```python
from build123d import *

# Parameters (mm, degrees)
PAD_DEPTH              = 66
SKETCH001_W            = 31.9
SKETCH001_H            = 39.95
PAD001_DEPTH           = 1
PAD002_DEPTH           = 1.2
PAD003_DEPTH           = 16
SKETCH011_W            = 16.471436
SKETCH011_H            = 30.415474
POCKET_DEPTH           = 5
POCKET001_DEPTH        = 8
POCKET002_DEPTH        = 5
LINEARPATTERN_COUNT    = 2
LINEARPATTERN_PITCH    = 32
POCKET003_DEPTH        = 31.901
LINEARPATTERN001_COUNT = 2
LINEARPATTERN001_PITCH = 28


with BuildPart() as part:
    # Sketch → Pad (new body)
    with BuildSketch(Plane.XY):
        Polygon((14.75, 37.75), (14.75, 0), (-14.75, 0), (-14.75, 37.75), (-12.25, 37.75), (-12.25, 38.75), (-15.95, 38.75), (-15.95, -1.2), (15.95, -1.2), (15.95, 38.75), (12.25, 38.75), (12.25, 37.75), align=None)
    extrude(amount=PAD_DEPTH)

    # Sketch001 (on Face13 of Pad) → Pad001 (join)
    with BuildSketch(Plane(origin=(0, 0, 0), x_dir=(1, 0, 0), z_dir=(0, 0, -1))):
        with Locations((0, -18.775)):
            Rectangle(SKETCH001_W, SKETCH001_H)
    extrude(amount=PAD001_DEPTH)

    # Sketch002 (on Face13 of Pad001) → Pad002 (join)
    with BuildSketch(Plane.XZ.offset(1.2)):
        Polygon((-15.95, 66), (-4, 94), (4, 94), (15.95, 66), align=None)
    extrude(amount=-PAD002_DEPTH)

    # Sketch007 (on Face8 of Pad002) → Pad003 (join)
    with BuildSketch(Plane(origin=(0, 0, 0), x_dir=(-1, 0, 0), z_dir=(0, 1, 0))):
        Polygon((-15.95, 66), (-14.7, 66), (-3.5, 88), (3.5, 88), (14.7, 66), (15.95, 66), (4, 94), (-4, 94), align=None)
    extrude(amount=PAD003_DEPTH)

    # Sketch011 (on Face24 of Pad003) → Pocket (cut)
    with BuildSketch(Plane(origin=(0, 0, -1), x_dir=(1, 0, 0), z_dir=(0, 0, -1))):
        with Locations((0, -31.207737)):
            Rectangle(SKETCH011_W, SKETCH011_H)
    extrude(amount=-POCKET_DEPTH, mode=Mode.SUBTRACT)

    # Sketch012 (on Face33 of Pocket) → Pocket001 (cut)
    with BuildSketch(Plane.XY.offset(94)):
        with BuildLine():
            ThreePointArc((2.985382, 13.549034), (-0.014618, 16.549034), (-3.014618, 13.549034))
            Line((-3.014618, 13.549034), (-3.014618, 11.03404))
            ThreePointArc((-3.014618, 11.03404), (-0.014618, 8.03404), (2.985382, 11.03404))
            Line((2.985382, 13.549034), (2.985382, 11.03404))
        make_face()
    extrude(amount=-POCKET001_DEPTH, mode=Mode.SUBTRACT)

    # Sketch014 (on Face30 of Pocket001) → Pocket002 (cut)
    with BuildSketch(Plane.XZ.offset(1.2)):
        Polygon((0, 25.833173), (-10.237929, 13.747521), (-10.237929, 5.434677), (10.297925, 5.434677), (10.297925, 13.443167), align=None)
    pocket002 = extrude(amount=-POCKET002_DEPTH, mode=Mode.SUBTRACT)

    # LinearPattern: Pocket002 ×2
    with Locations(*[(0, 0, i * LINEARPATTERN_PITCH) for i in range(1, LINEARPATTERN_COUNT)]):
        add(pocket002, mode=Mode.SUBTRACT)

    # Sketch015 (on Face29 of LinearPattern) → Pocket003 (cut, through all)
    with BuildSketch(Plane.YZ.offset(15.95)):
        Polygon((18.770079, 31.374571), (6.687755, 18.189028), (6.687755, 5.829207), (30.620473, 5.829207), (30.620473, 18.442136), align=None)
    pocket003 = extrude(amount=-POCKET003_DEPTH, mode=Mode.SUBTRACT)

    # LinearPattern001: Pocket003 ×2
    with Locations(*[(0, 0, i * LINEARPATTERN001_PITCH) for i in range(1, LINEARPATTERN001_COUNT)]):
        add(pocket003, mode=Mode.SUBTRACT)


solid = part.part
```
Geometry: final body of the model. Coordinates: model frame, mm. A direction names the side the tool comes from. Round coordinates to 2 decimals unless told otherwise and drop trailing zeros. Order: outer loops, then holes, each group sorted by start corner. A loop starts at its lowest first (then second) coordinate and runs counter-clockwise, first axis right, second up. Notation, with made-up numbers: M 44,27 L 51,27 A32 cw 51,60 Z; hole C 82.5,74 d7. An arc over 180 degrees is marked long. Use one line per item in the form item = value. Start each with the question number.
Q1. Cut plane B-B (y = 4). Return loops of the section in (x, z), and give its area (4 significant figures).
Q2. Material intervals for line 1 (X direction, y = 13, z = 58); line 2 (Z direction, x = -13, y = 34.5); line 3 (Y direction, x = -2, z = 75), sorted ascending. Write a range as [from, to].
Q3. Mould query, pull axis Z, two halves, no side actions, for faces 5 (the face through (0, 14, -1)), 6 (the face through (-0.081, 8.035, 91.042)), 7 (the face through (-15.342, 24.778, 52.818)). Classes: +Z half, -Z half, draft (parallel to the pull), parting line (faces both ways), or undercut.
Q4. Cut plane A-A (y = 33.5). Return loops of the section in (x, z), and give its area (3 significant figures).
Q5. Access query for faces 1 (the face through (5.22, -0.61, 51.55)), 2 (the face through (-15.34, 12.81, 24.87)), 3 (the face through (2.66, 14.91, 91.04)), 4 (the face through (9.2, 7.9, 76.8)). Directions: +Z, -Z, +X, -X, +Y, -Y. A direction counts if a zero-diameter tool reaches every point of the face in a straight line with its end or side. Return the directions, or none.
Q6. Pin query (flat end, axial travel): pin 1 Ø3 at (y, z) = (12.5, 91.5) entering from -X; pin 2 Ø4 at (x, y) = (9, 13) entering from +Z; pin 3 Ø2 at (y, z) = (12, 90) entering from +X; pin 4 Ø1.5 at (y, z) = (29.5, 42) entering from +X. Return the tip coordinate at first contact, or that it passes through.
Q7. Cut plane D-D (x = -6). Return loops of the section in (y, z), and give its area (3 significant figures).
Q8. Cut plane C-C (z = 10.5). Return loops of the section in (x, y).
Geometry results:
q1.outline = M -15.95,-1 L 15.95,-1 L 15.95,66 L 4,94 L -4,94 L -15.95,66 Z; hole M -14.75,0 L 14.75,0 L 14.75,66 L 14.7,66 L 3.5,88 L -3.5,88 L -14.7,66 L -14.75,66 Z
q1.area = 348.5 mm^2
q2.line_1 = [-15.95, -14.75], [14.75, 15.95]
q2.line_2 = [-1, 0]
q2.line_3 = [-1.2, 0]
q3.face_5 = -Z half
q3.face_6 = draft
q3.face_7 = undercut
q4.outline = M -15.95,-1 L -8.24,-1 L -8.24,0 L -14.75,0 L -14.75,66 L -15.95,66 Z; M 8.24,-1 L 15.95,-1 L 15.95,66 L 14.75,66 L 14.75,0 L 8.24,0 Z
q4.area = 174 mm^2
q5.face_1 = +Y, -Y
q5.face_2 = +X, -X
q5.face_3 = +Z
q5.face_4 = +Y
q6.pin_1 = -5.71
q6.pin_2 = 86.97
q6.pin_3 = 6.13
q6.pin_4 = through
q7.outline = M -1.2,-1 L 16,-1 L 16,0 L 0,0 L 0,5.43 L -1.2,5.43 Z; M -1.2,18.75 L 0,18.75 L 0,37.43 L -1.2,37.43 Z; M -1.2,50.75 L 0,50.75 L 0,83.09 L 16,83.09 L 16,89.31 L -1.2,89.31 Z
q7.area = 192 mm^2
q8.outline = M -15.95,-1.2 L -10.24,-1.2 L -10.24,0 L -14.75,0 L -14.75,6.69 L -15.95,6.69 Z; M -15.95,30.62 L -14.75,30.62 L -14.75,37.75 L -12.25,37.75 L -12.25,38.75 L -15.95,38.75 Z; M 10.3,-1.2 L 15.95,-1.2 L 15.95,6.69 L 14.75,6.69 L 14.75,0 L 10.3,0 Z; M 12.25,37.75 L 14.75,37.75 L 14.75,30.62 L 15.95,30.62 L 15.95,38.75 L 12.25,38.75 Z
